Design review of the part built by this model. Coordinates are the model's own, in mm. Face numbers are marked on the shaded views. A direction names the side the tool comes from. Give positions to 0.01 mm unless a question says otherwise; leave off trailing zeros. Loops run counter-clockwise (first coordinate to the right, second up) from the corner with the lowest first, then second, coordinate; pieces in that order, holes last. Notation, with made-up numbers: M -17.5,68.25 L 20.5,68.25 A19 ccw 20.5,92.25 Z; hole C -22.5,-1.75 d6. An arc over 180 degrees is marked long. Answer as CSV lines item,"result".
```python
from build123d import *

# Parameters (mm, degrees)
SKETCH1_R           = 10
BOSS_EXTRUDE1_DEPTH = 10
FILLET1_R           = 1.5


with BuildPart() as part:
    # Sketch1 → Boss-Extrude1 (new, symmetric)
    with BuildSketch(Plane(origin=(0, 0, 0), x_dir=(1, 0, 0), z_dir=(0, 1, 0))):
        with BuildLine():
            Line((0, 25), (180, 25))
            ThreePointArc((180, 25), (205, 0), (180, -25))
            Line((180, -25), (0, -25))
            ThreePointArc((0, -25), (-25, 0), (0, 25))
        make_face()
        with Locations(Location((0, 0, 0), (0, 0, 270))):
            Circle(SKETCH1_R, mode=Mode.SUBTRACT)
        with BuildLine():
            Line((30, 7.5), (180, 7.5))
            ThreePointArc((180, 7.5), (187.5, 0), (180, -7.5))
            Line((180, -7.5), (30, -7.5))
            ThreePointArc((30, -7.5), (22.5, 0), (30, 7.5))
        make_face(mode=Mode.SUBTRACT)
    extrude(amount=BOSS_EXTRUDE1_DEPTH, both=True)

    # Fillet1
    fillet1_edges = [part.edges().sort_by_distance(p)[0] for p in [
        (205, 10, 0),
        (90, 10, -25),
        (-25, 10, 0),
        (90, -10, -25),
        (205, -10, 0),
        (90, -10, 25),
        (-25, -10, 0),
        (90, 10, 25),
    ]]
    fillet(fillet1_edges, radius=FILLET1_R)


solid = part.part
```
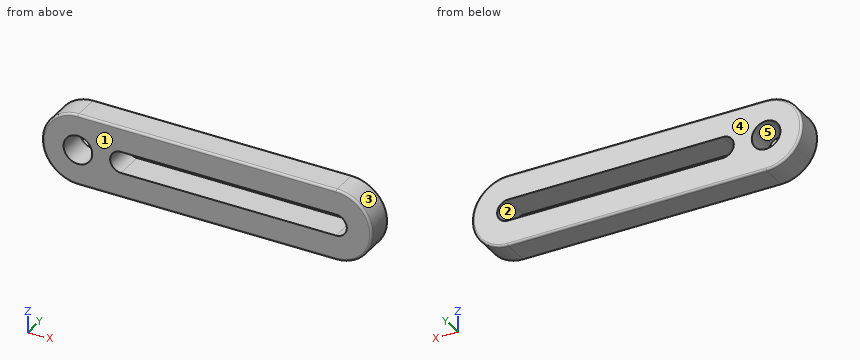
1. To check wall thickness, follow L1, parallel to X at y = 4.5, z = 0; L2, parallel to X at y = 8.25, z = 5.5; L3, parallel to Z at x = 44.5, y = 6. State the ranges of each line that lie inside material, in increasing order. Write a range as [from, to].
Answer block:
L1,"[-25, -10], [10, 22.5], [187.5, 205]"
L2,"[-24.39, -8.35], [8.35, 24.9], [185.1, 204.39]"
L3,"[-25, -7.5], [7.5, 25]"
2. The part is to be moulded in two halves that separate along Z. For the marked faces 3, 4 and 5, say which applies: pulls with the +Z half, pulls with the -Z half, needs draft (parallel to the pull), parting line crosses it, or undercut.
Answer block:
face 3,"parting line crosses it"
face 4,"needs draft"
face 5,"undercut"
3. We need section A-A, the plane x = 140.5. Write out the cut boundary in (y, z).
Answer block:
outline,"M -10,-23.5 A1.5 ccw -8.5,-25 L 8.5,-25 A1.5 ccw 10,-23.5 L 10,-7.5 L -10,-7.5 Z; M -10,7.5 L 10,7.5 L 10,23.5 A1.5 ccw 8.5,25 L -8.5,25 A1.5 ccw -10,23.5 Z"
4. We need section C-C, the plane y = -0.5. Write out the cut boundary in (x, z), plus the area to 3 significant figures.
Answer block:
outline,"M 0,-25 L 180,-25 A25 ccw 180,25 L 0,25 A25 ccw Z; hole C 0,0 d20; hole M 30,-7.5 L 180,-7.5 A7.5 ccw 180,7.5 L 30,7.5 A7.5 ccw Z"
area,"8,220 mm²"
5. For the marked faces 1 and 2, list the 3-axis set-ups (+Z, -Z, +X, -X, +Y, -Y) from which the entire face can be reached by the end or side of a thin tool; tool diameter is ignored.
Answer block:
face 1,"+Z, -Z, +X, -X, -Y"
face 2,"+Y, -Y"
6. We need section B-B, the plane z = 0. Write out the cut boundary in (x, y), plus the area to 3 significant figures.
Answer block:
outline,"M -25,-8.5 A1.5 ccw -23.5,-10 L -10,-10 L -10,10 L -23.5,10 A1.5 ccw -25,8.5 Z; M 10,-10 L 22.5,-10 L 22.5,10 L 10,10 Z; M 187.5,-10 L 203.5,-10 A1.5 ccw 205,-8.5 L 205,8.5 A1.5 ccw 203.5,10 L 187.5,10 Z"
area,"898 mm²"
7. For P1, Ø8, axis at y = -4.5, z = -9.5, coming from the -X side; P2, Ø12, axis at y = 1.5, z = -17, coming from the +X side; P3, Ø10, axis at y = -3.5, z = -5, coming from the +X side, all flat-tipped, find the tip position at first contact; note any pin that passes through.
Answer block:
P1,"x = -24.39"
P2,"x = 202.45"
P3,"x = 205"
